The listing builds one solid part. Answer for the finished solid, in the listing's coordinates (mm). Face numbers are marked on the shaded views. A direction names the side the tool comes from. Round coordinates to 2 decimals unless told otherwise and drop trailing zeros. Loops run counter-clockwise (first coordinate to the right, second up) from the corner with the lowest first, then second, coordinate; pieces in that order, holes last. Notation, with made-up numbers: M 6,9.25 L 24,9.25 A9 ccw 24,24.25 Z; hole C 3.5,32 d8. An arc over 180 degrees is marked long. Answer as a JSON object with one key per item and string values.
Autodesk Inventor part; units mm, degrees
ref_plane "YZ Plane" through (0, 0, 0) normal (1, 0, 0) x (0, 1, 0)
ref_plane "XZ Plane" through (0, 0, 0) normal (0, 1, 0) x (-1, 0, 0)
ref_plane "XY Plane" through (0, 0, 0) normal (0, 0, 1) x (1, 0, 0)
sketch "Sketch1" plane through (0, 0, 0) normal (0, 1, 0) x (-1, 0, 0)
  line L0 (0, 0) -> (-58, 0)
  line L1 (-58, 0) -> (-58, -41)
  line L2 (-58, -41) -> (0, -41)
  line L3 (0, -41) -> (0, 0)
  line L4 (-45.5, -30) -> (-52.5, -30)
  line L5 (-52.5, -30) -> (-52.5, -11.5)
  line L6 (-52.5, -11.5) -> (-45.5, -11.5)
  line L7 (-45.5, -11.5) -> (-45.5, -30)
  dimension "d0" = 58
  dimension "d1" = 41
  dimension "d2" = 11.5
  dimension "d3" = 11
  dimension "d4" = 7
  dimension "d5" = 5.5
extrude "Extrusion1" add sketch "Sketch1" along normal blind 4
sketch "Sketch2" plane through (0, 4, 0) normal (0, 1, 0) x (1, 0, 0)
  line L0 (45.5, 11.5) -> (45.5, 30)
  line L1 (45.5, 30) -> (52.5, 30)
  line L2 (52.5, 30) -> (52.5, 11.5)
  line L3 (52.5, 11.5) -> (45.5, 11.5)
  line L4 (54, 31.5) -> (44, 31.5)
  line L5 (44, 31.5) -> (44, 10)
  line L6 (44, 10) -> (54, 10)
  line L7 (54, 10) -> (54, 31.5)
  point P0 (0, 0)
  dimension "d8" = 1.5
extrude "Extrusion2" add sketch "Sketch2" along normal blind 21
sketch "Sketch3" plane through (0, 4, 0) normal (0, 1, 0) x (1, 0, 0)
  line L0 (58, 41) -> (0, 41) construction
  line L1 (0, 41) -> (0, 0) construction
  line L2 (0, 0) -> (58, 0) construction
  line L3 (58, 0) -> (58, 41) construction
  line L4 (4, 37) -> (54, 37) construction
  line L5 (54, 37) -> (54, 4) construction
  line L6 (54, 4) -> (4, 4) construction
  line L7 (4, 4) -> (4, 37) construction
  line L8 (0, 20.5) -> (58, 20.5) construction
  line L9 (29, 0) -> (29, 41) construction
  line L10 (0, 16.5) -> (4, 16.5)
  line L11 (4, 16.5) -> (4, 20.5)
  line L12 (0, 16.5) -> (0, 20.5)
  line L13 (0, 8.5) -> (4, 8.5)
  line L14 (4, 8.5) -> (4, 4)
  line L15 (4, 4) -> (9, 4)
  line L16 (9, 4) -> (9, 0)
  line L17 (9, 0) -> (0, 0)
  line L18 (0, 0) -> (0, 8.5)
  line L19 (17, 4) -> (17, 0)
  line L20 (17, 0) -> (25, 0)
  line L21 (25, 0) -> (25, 4)
  line L22 (25, 4) -> (17, 4)
  line L23 (0, 24.5) -> (4, 24.5)
  line L24 (4, 24.5) -> (4, 20.5)
  line L25 (0, 24.5) -> (0, 20.5)
  line L26 (0, 32.5) -> (4, 32.5)
  line L27 (4, 32.5) -> (4, 37)
  line L28 (4, 37) -> (9, 37)
  line L29 (9, 37) -> (9, 41)
  line L30 (9, 41) -> (0, 41)
  line L31 (0, 41) -> (0, 32.5)
  line L32 (17, 37) -> (17, 41)
  line L33 (17, 41) -> (25, 41)
  line L34 (25, 41) -> (25, 37)
  line L35 (25, 37) -> (17, 37)
  line L36 (58, 41) -> (58, 0) construction
  line L37 (54, 4) -> (54, 37) construction
  line L38 (58, 16.5) -> (54, 16.5)
  line L39 (54, 16.5) -> (54, 20.5)
  line L40 (58, 16.5) -> (58, 20.5)
  line L41 (58, 8.5) -> (54, 8.5)
  line L42 (54, 8.5) -> (54, 4)
  line L43 (54, 4) -> (49, 4)
  line L44 (49, 4) -> (49, 0)
  line L45 (49, 0) -> (58, 0)
  line L46 (58, 0) -> (58, 8.5)
  line L47 (41, 4) -> (41, 0)
  line L48 (41, 0) -> (33, 0)
  line L49 (33, 0) -> (33, 4)
  line L50 (33, 4) -> (41, 4)
  line L51 (49, 37) -> (49, 41)
  line L52 (54, 24.5) -> (54, 20.5)
  line L53 (54, 32.5) -> (54, 37)
  line L54 (54, 37) -> (49, 37)
  line L55 (58, 24.5) -> (58, 20.5)
  line L56 (58, 24.5) -> (54, 24.5)
  line L57 (58, 32.5) -> (54, 32.5)
  line L58 (58, 41) -> (58, 32.5)
  line L59 (49, 41) -> (58, 41)
  line L60 (41, 37) -> (41, 41)
  line L61 (33, 37) -> (41, 37)
  line L62 (41, 41) -> (33, 41)
  line L63 (33, 41) -> (33, 37)
  dimension "d11" = 4
  dimension "d12" = 4
  dimension "d13" = 8
  dimension "d14" = 8
  dimension "d15" = 4
  dimension "d16" = 8
extrude "Extrusion3" cut sketch "Sketch3" against normal up to surface (4 mm away)
properties part number "top" material "PBT Plastic Black"
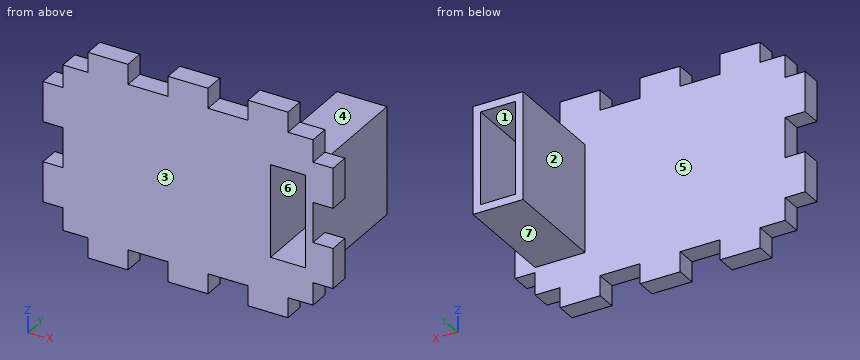
Item 1: Which of the six approach directions +Z, -Z, +X, -X, +Y, -Y give full straight-line access (tool end or side, diameter ignored) to the marked faces 1, 2 and 3?
Values follow:
{"face 1": "+Y, -Y", "face 2": "+Z, -Z, -X, +Y", "face 3": "+Z, -Z, +X, -X, -Y"}
Item 2: The part is cut by section A-A (x = 48). Give the vertices of the cut face in (y, z), then the cut area to 3 significant figures.
Values follow:
{"outline": "M 0,-41 L 4,-41 L 4,-31.5 L 25,-31.5 L 25,-30 L 0,-30 Z; M 0,-11.5 L 25,-11.5 L 25,-10 L 4,-10 L 4,0 L 0,0 Z", "area": "153 mm^2"}
Item 3: The part is cut by section B-B (z = -21.5). Give the vertices of the cut face in (x, y).
Values follow:
{"outline": "M 4,0 L 45.5,0 L 45.5,25 L 44,25 L 44,4 L 4,4 Z; M 52.5,0 L 54,0 L 54,25 L 52.5,25 Z"}
Item 4: Straight lines are drawn through the part: line 1 (X direction, y = 19.75, z = -26); line 2 (Z direction, x = 48, y = 3.75); line 3 (X direction, y = 21.5, z = -11). For each, find the intervals that lie inside material, in ascending order.
Values follow:
{"line 1": "44 to 45.5, 52.5 to 54", "line 2": "-41 to -30, -11.5 to 0", "line 3": "44 to 54"}
Item 5: The part is cut by section C-C (y = 20.75). Give the vertices of the cut face in (x, z).
Values follow:
{"outline": "M 44,-31.5 L 54,-31.5 L 54,-10 L 44,-10 Z; hole M 45.5,-30 L 52.5,-30 L 52.5,-11.5 L 45.5,-11.5 Z"}
Item 6: Determine the mould class of the marked faces 4, 5, 6 and 7 for opening direction Z: released by +Z, released by -Z, zero draft, split by the parting line, or undercut.
Values follow:
{"face 4": "released by +Z", "face 5": "zero draft", "face 6": "undercut", "face 7": "released by -Z"}
Item 7: Flat-ended cylindrical pins translate along their axes: P1, Ø1.5, axis at x = 22, y = 4.5, coming from the +Z side; P2, Ø4.5, axis at y = 2, z = -1, coming from the +X side; P3, Ø2, axis at x = 56, y = 2, coming from the -Z side. Find the tip coordinate at first contact, or state that the pin passes through.
Values follow:
{"P1": "z = -4", "P2": "x = 49", "P3": "z = -32.5"}
Item 8: The part is cut by section D-D (z = -15). Give the vertices of the cut face in (x, y).
Values follow:
{"outline": "M 0,0 L 45.5,0 L 45.5,25 L 44,25 L 44,4 L 0,4 Z; M 52.5,0 L 58,0 L 58,4 L 54,4 L 54,25 L 52.5,25 Z"}
